Work out the finished part from the listing and answer in its coordinate system (mm). Give positions to 0.01 mm unless a question says otherwise; leave off trailing zeros. Order: outer loops, then holes, each group sorted by start corner. A loop starts at its lowest first (then second) coordinate and runs counter-clockwise, first axis right, second up. Notation, with made-up numbers: (39, 39.25) - (75, 39.25) arc R21 cw to (75, 44.25) - close; hole circle Ø5 at (33.25, 88.5). An arc over 180 degrees is marked (long way). Put each result on its own line as item: value.
```python
from build123d import *

# Parameters (mm, degrees)
SKETCH2_R                    = 12.7
BOSS_EXTRUDE1_DEPTH          = 34.925
F_3_8_0_375_DIAMETER_HOLE1_D = 9.525
F_1_8_0_125_DIAMETER_HOLE1_D = 3.175


with BuildPart() as part:
    # Sketch1 → Revolve1 (revolve)
    with BuildSketch(Plane.XY, mode=Mode.PRIVATE) as revolve1_sk:
        Polygon((0, 0), (0, 38.1), (-8.796078082, 0), align=None)
    revolve(revolve1_sk.sketch.rotate(Axis((0, 0, 0), (0, 1, 0)), 270), axis=Axis((0, 0, 0), (0, 1, 0)))


with BuildPart() as body_2:
    # Sketch2 → Boss-Extrude1 (new body)
    with BuildSketch(Plane.XZ):
        with Locations(Location((0, 0, 0), (0, 0, 270))):
            Circle(SKETCH2_R)
    extrude(amount=-BOSS_EXTRUDE1_DEPTH)

    # Combine1: cut part
    add(part.part, mode=Mode.SUBTRACT)

    # 3/8 (0.375) Diameter Hole1 (through all)
    with Locations(Plane(origin=(0, 34.925, 0), x_dir=(1, 0, 0), z_dir=(0, 1, 0))):
        with Locations((0, 0)):
            Hole(F_3_8_0_375_DIAMETER_HOLE1_D / 2)

    # 1/8 (0.125) Diameter Hole1 (through all)
    with Locations(Plane(origin=(0, 0, 0), x_dir=(1, 0, 0), z_dir=(0, -0.7071067811865475, 0.7071067811865477))):
        with Locations((0, 29.466465397)):
            Hole(F_1_8_0_125_DIAMETER_HOLE1_D / 2)


solid = body_2.part
```
(1) Section D-D, the plane y = 32 is taken. Count the separate pieces of the cut face and the enclosed holes in it, then the cut area to 3 significant figures.
Geometry check:
separate pieces: 1
enclosed holes: 2
area: 424 mm²
(2) Section C-C, the plane x = 9.5 is taken. Write down the section's boundary in (y, z) (3 decimals), then the cut area to 3 significant figures.
Geometry check:
outline: (0, -8.429) - (34.925, -8.429) - (34.925, 8.429) - (0, 8.429) - close
area: 589 mm²
(3) Section A-A, the plane z = 0 is taken. Write down the section's boundary in (x, y) (1 decimal), then the cut area to 3 significant figures.
Geometry check:
outline: (-12.7, 0) - (-8.8, 0) - (-4.8, 17.5) - (-4.8, 34.9) - (-12.7, 34.9) - close; (4.8, 17.5) - (8.8, 0) - (12.7, 0) - (12.7, 34.9) - (4.8, 34.9) - close
area: 484 mm²
(4) Section B-B, the plane x = 0 is taken. Write down the section's boundary in (y, z) (1 decimal), then the cut area to 3 significant figures.
Geometry check:
outline: (0, -12.7) - (34.9, -12.7) - (34.9, -4.8) - (17.5, -4.8) - (0, -8.8) - close; (0, 8.8) - (17.5, 4.8) - (34.7, 4.8) - (26.7, 12.7) - (0, 12.7) - close; (31.2, 12.7) - (34.9, 9) - (34.9, 12.7) - close
area: 457 mm²
(5) Determine the mould class of faces 1 (the face through (0, 34.925, -5)), 2 (the face through (9, 0, -3)), 3 (the face through (0.34, 30.86, 8.62)) for opening direction Y: pulls with the +Y half, pulls with the -Y half, needs draft (parallel to the pull), parting line crosses it, or undercut.
Geometry check:
face 1: pulls with the +Y half
face 2: pulls with the -Y half
face 3: undercut
(6) Straight lines are drawn through the part: line 1 (Z direction, x = 0, y = 26.25); line 2 (Z direction, x = -3, y = 24); line 3 (Y direction, x = 1.25, z = 10) (3 decimals). For each, find the intervals that lie inside material, in ascending order.
Geometry check:
line 1: z = -12.7 to -4.76, 4.76 to 12.7
line 2: z = -12.34 to -3.7, 3.7 to 12.34
line 3: y = 0 to 30.288, 33.056 to 34.925
